```python
from build123d import *

# Parameters (mm, degrees)
F1_DEPTH = 15.875
F3_D     = 6.35


with BuildPart() as f1:
    # F0 (on Front) → F1 (new body)
    with BuildSketch(Plane.XZ):
        with BuildLine():
            Line((-39.947468, -18.41737), (-26.839392, -18.41737))
            ThreePointArc((-26.839392, -18.41737), (-8.197468, 3.58263), (10.444455, -18.41737))
            Line((10.444455, -18.41737), (23.552532, -18.41737))
            Line((23.552532, -18.41737), (23.552532, -17.14737))
            Line((23.552532, -17.14737), (11.887384, -17.14737))
            ThreePointArc((11.887384, -17.14737), (-8.197468, 4.85263), (-28.282321, -17.14737))
            Line((-28.282321, -17.14737), (-39.947468, -17.14737))
            Line((-39.947468, -17.14737), (-39.947468, -18.41737))
        make_face()
    extrude(amount=F1_DEPTH)

    # F3 (through all)
    with Locations(Plane(origin=(0, 0, -18.41737), x_dir=(1, 0, 0), z_dir=(0, 0, -1))):
        with Locations((-33.597468, 7.9375), (17.202532, 7.9375)):
            Hole(F3_D / 2)


solid = f1.part
```
Verification items for the finished model (mm, model axes). Round coordinates to 2 decimals unless told otherwise and drop trailing zeros. Order: outer loops, then holes, each group sorted by start corner. A loop starts at its lowest first (then second) coordinate and runs counter-clockwise, first axis right, second up. Notation, with made-up numbers: (34.25, 49) -> (47.25, 49) arc R23 ccw to (47.25, 83) -> close; hole circle Ø1 at (51, -26). An arc over 180 degrees is marked (long way). Put each result on its own line as item: value. Start each with the question number.
(1) Depth check by flat-ended pin: pin 1 Ø1.5 at (y, z) = (-5, -15) entering from -X; pin 2 Ø1.5 at (x, y) = (-24, -5) entering from -Z; pin 3 Ø1 at (x, z) = (-23.5, -2) entering from +Y; pin 4 Ø9.5 at (x, y) = (20.5, -6) entering from +Z. Enter the tip coordinate at first touch or a pass-through.
(2) Draft check along Z on faces 1 (the face through (-39.947, -8, -18)), 2 (the face through (14, -6, -18.417)), 3 (the face through (-8.657, -7.826, 3.577)). Enter one of: +Z half, -Z half, draft (parallel to the pull), parting line (faces both ways), or undercut.
(3) Section check A-A (z = -11.5). Enter the section's corners in (x, y) (3 decimals), then the cut area to 3 significant figures.
(4) Section check C-C (y = -3). Enter the section's corners in (x, z), then the cut area to 3 significant figures.
(5) Material ranges on line 1 along Z through (x, y) = (14.5, -11.5); line 2 along X through (y, z) = (-9, -7); line 3 along X through (y, z) = (-5.75, -4.25), recorded low to high.
(6) Section check D-D (z = -8). Enter the section's corners in (x, y) (3 decimals).
(7) Section check B-B (y = -6.75). Enter the section's corners in (x, z), then the cut area to 3 significant figures.
Completed:
1. pin 1: stops at x = -28.37
1. pin 2: stops at z = -6.2
1. pin 3: stops at y = 0
1. pin 4: stops at z = -17.15
2. face 1: draft
2. face 2: -Z half
2. face 3: undercut
3. outline: (-28.001, -15.875) -> (-26.706, -15.875) -> (-26.706, 0) -> (-28.001, 0) -> close; (10.312, -15.875) -> (11.607, -15.875) -> (11.607, 0) -> (10.312, 0) -> close
3. area: 41.1 mm2
4. outline: (-39.95, -18.42) -> (-26.84, -18.42) arc R18.9 cw (long way) to (10.44, -18.42) -> (23.55, -18.42) -> (23.55, -17.15) -> (11.89, -17.15) arc R20.17 ccw (long way) to (-28.28, -17.15) -> (-39.95, -17.15) -> close
4. area: 116 mm2
5. line 1: z = -18.42 to -17.15
5. line 2: x = -26.57 to -25.17, 8.77 to 10.18
5. line 3: x = -25.06 to -23.52, 7.12 to 8.66
6. outline: (-26.992, -15.875) -> (-25.622, -15.875) -> (-25.622, 0) -> (-26.992, 0) -> close; (9.227, -15.875) -> (10.597, -15.875) -> (10.597, 0) -> (9.227, 0) -> close
7. outline: (-39.95, -18.42) -> (-36.54, -18.42) -> (-36.54, -17.15) -> (-39.95, -17.15) -> close; (-30.65, -18.42) -> (-26.84, -18.42) arc R18.9 cw (long way) to (10.44, -18.42) -> (14.26, -18.42) -> (14.26, -17.15) -> (11.89, -17.15) arc R20.17 ccw (long way) to (-28.28, -17.15) -> (-30.65, -17.15) -> close; (20.15, -18.42) -> (23.55, -18.42) -> (23.55, -17.15) -> (20.15, -17.15) -> close
7. area: 101 mm2
